Check sheet for the modelled part. Datum: model origin and axes. Units: mm. A direction names the side the tool comes from. Give positions to 0.01 mm unless a question says otherwise; leave off trailing zeros. Loops run counter-clockwise (first coordinate to the right, second up) from the corner with the lowest first, then second, coordinate; pieces in that order, holes last. Notation, with made-up numbers: (9, -24) - (60, -24) arc R25 cw to (60, -5) - close; hole circle Ø2 at (36, 24.5). An arc over 180 degrees is marked (long way). Answer in a Markdown table with one row per item. Add a question column.
(1) Sectioned sample at A-A on y = 40.75. Enter the section's corners in (x, z), then the cut area to 3 significant figures.
(2) Set-up check for faces 1 (the face through (-0.937, 39.675, 21.183)), 2 (the face through (5, 33.783, 22)), 3 (the face through (1, 42, 22)): record each of +Z, -Z, +X, -X, +Y, -Y from which the full face is reachable in a straight line by a thin tool's end or side.
(3) Sectioned sample at B-B on x = 6. Enter the section's corners in (y, z).
(4) Sectioned sample at C-C on z = 19.75. Enter the section's corners in (x, y), then the cut area to 3 significant figures.
(5) Sectioned sample at D-D on z = 21.5. Enter the section's corners in (x, y).
(6) Draft check along Z on faces 4 (the face through (5, 42, 17.943)), 5 (the face through (5, 49.783, 22)), 6 (the face through (5, 48.183, 22)), 7 (the face through (5, 42, 25.943)). Enter one of: released by +Z, released by -Z, zero draft, split by the parting line, or undercut.
(7) Thickness scan on L1, parallel to Y at x = 4.5, z = 24; L2, parallel to Z at x = 2.25, y = 43; L3, parallel to X at y = 35.25, z = 21.75. Record the ranges inside material, lowest first.
from build123d import *

# Parameters (mm, degrees)
F0_W     = 16
F0_H     = 8
F1_DEPTH = 9.5
F2_R     = 1.25
F3_DEPTH = 1.9
F4_W     = 12.8
F4_H     = 4.8
F6_DEPTH = 8.5


# Not quite as in the source:
# - a feature names something its author has since deleted; it is built from what else it names


with BuildPart() as f1:
    # F0 (on Right) → F1 (new body)
    with BuildSketch(Plane.YZ):
        with Locations((41.7828243226, 21.9434328547)):
            Rectangle(F0_W, F0_H)
    extrude(amount=F1_DEPTH)

    # F2 (on face) → F3 (join)
    with BuildSketch(Plane(origin=(0, 0, 0), x_dir=(0, -1, 0), z_dir=(-1, 0, 0))):
        with Locations((-44.8828243226, 21.9434328547)):
            Circle(F2_R)
        with Locations((-38.6828243226, 21.9434328547)):
            Circle(F2_R)
    extrude(amount=F3_DEPTH)

    # F4 (on face) → F6 (cut)
    with BuildSketch(Plane.YZ.offset(9.5)):
        with Locations((41.7828243226, 21.9434328547)):
            Rectangle(F4_W, F4_H)
    extrude(amount=-F6_DEPTH, mode=Mode.SUBTRACT)


solid = f1.part
Reply:
| question | item | result |
|---|---|---|
| 1 | outline | (0, 17.94) - (9.5, 17.94) - (9.5, 19.54) - (1, 19.54) - (1, 24.34) - (9.5, 24.34) - (9.5, 25.94) - (0, 25.94) - close |
| 1 | area | 35.2 mm^2 |
| 2 | face 1 | -X |
| 2 | face 2 | +Z, -Z, +X, -X, -Y |
| 2 | face 3 | +X |
| 3 | outline | (33.78, 17.94) - (49.78, 17.94) - (49.78, 25.94) - (33.78, 25.94) - close; hole (35.38, 19.54) - (48.18, 19.54) - (48.18, 24.34) - (35.38, 24.34) - close |
| 4 | outline | (0, 33.78) - (9.5, 33.78) - (9.5, 35.38) - (1, 35.38) - (1, 48.18) - (9.5, 48.18) - (9.5, 49.78) - (0, 49.78) - close |
| 4 | area | 43.2 mm^2 |
| 5 | outline | (-1.9, 37.51) - (0, 37.51) - (0, 33.78) - (9.5, 33.78) - (9.5, 35.38) - (1, 35.38) - (1, 48.18) - (9.5, 48.18) - (9.5, 49.78) - (0, 49.78) - (0, 46.05) - (-1.9, 46.05) - (-1.9, 43.71) - (0, 43.71) - (0, 39.85) - (-1.9, 39.85) - close |
| 6 | face 4 | released by -Z |
| 6 | face 5 | zero draft |
| 6 | face 6 | undercut |
| 6 | face 7 | released by +Z |
| 7 | L1 | 33.78 to 35.38, 48.18 to 49.78 |
| 7 | L2 | 17.94 to 19.54, 24.34 to 25.94 |
| 7 | L3 | 0 to 9.5 |
